Check sheet for the modelled part. Datum: model origin and axes. Units: mm. Face numbers are marked on the shaded views. Coordinates: 2 decimals unless noted, no trailing zeros. Loops run counter-clockwise (first coordinate to the right, second up) from the corner with the lowest first, then second, coordinate; pieces in that order, holes last. Notation, with made-up numbers: M 73,89 L 77,89 A16 ccw 77,103 Z; hole C 59,-2 d10. An arc over 180 degrees is marked long. Answer as CSV lines item,"result". Start each with the question number.
from build123d import *

# Parameters (mm, degrees)
F0_R     = 14.2875
F0_R_2   = 7.9375
F1_DEPTH = 4.7625
F2_R     = 1.190625
F3_DEPTH = 25.4
F5_DEPTH = 19.05


with BuildPart() as f1:
    # F0 (on Top) → F1 (new body)
    with BuildSketch(Plane.XY):
        Circle(F0_R)
        Circle(F0_R_2, mode=Mode.SUBTRACT)
    extrude(amount=F1_DEPTH)

    # F2 (on Top) → F3 (cut)
    with BuildSketch(Plane.XY):
        with Locations((0, 11.1125)):
            Circle(F2_R)
        with Locations((11.1125, 0)):
            Circle(F2_R)
        with Locations((-11.1125, 0)):
            Circle(F2_R)
        with Locations((0, -11.1125)):
            Circle(F2_R)
    extrude(amount=F3_DEPTH, mode=Mode.SUBTRACT)

    # F4 (on Top) → F5 (join)
    with BuildSketch(Plane.XY):
        with BuildLine():
            Line((5.61266, 5.61266), (12.347852, 12.347852))
            ThreePointArc((12.347852, 12.347852), (11.176734, 13.417135), (9.91344, 14.375765))
            Line((9.91344, 14.375765), (2.91897, 7.381295))
            ThreePointArc((2.91897, 7.381295), (4.356512, 6.635112), (5.61266, 5.61266))
        make_face()
        with BuildLine():
            Line((7.381295, 2.91897), (14.375765, 9.91344))
            ThreePointArc((14.375765, 9.91344), (13.417135, 11.176734), (12.347852, 12.347852))
            Line((12.347852, 12.347852), (5.61266, 5.61266))
            ThreePointArc((5.61266, 5.61266), (6.635112, 4.356512), (7.381295, 2.91897))
        make_face()
    extrude(amount=F5_DEPTH)


solid = f1.part
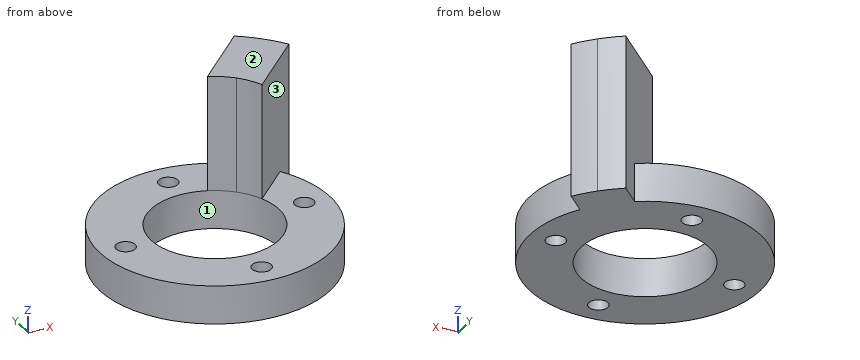
Item 1: Sectioned sample at B-B, the plane x = -3.5. Record the boundary of the cut face in (y, z).
Item 2: Release check for a two-part mould opening along X. For the marked faces 1, 2 and 3 record: released by +X, released by -X, zero draft, split by the parting line, or undercut.
Item 3: Material ranges on line 1 (X direction, y = 0, z = 1.3); line 2 (Z direction, x = -12.25, y = 0.75), recorded low to high. Write a range as from..to.
Item 4: Go/stop test with flat-tipped pins: pin 1 (2 mm diameter, centred on y = 6.5, z = 17, fed in from +X); pin 2 (1.9 mm diameter, centred on x = 0, y = 11.11, fed in from -Z); pin 3 (2 mm diameter, centred on y = 8, z = 5.5, fed in from +X); pin 4 (2.5 mm diameter, centred on x = 11.11, y = 0, fed in from +Z). Record where each tip stops, or that it passes through.
Item 5: Sectioned sample at D-D, the plane z = 15.5. Record the boundary of the cut face in (x, y).
Item 6: Sectioned sample at A-A, the plane y = 0. Record the boundary of the cut face in (x, z).
Reply:
1,outline,"M -13.85,0 L -7.12,0 L -7.12,4.76 L -13.85,4.76 Z; M 7.12,0 L 13.85,0 L 13.85,4.76 L 7.12,4.76 Z"
2,face 1,"undercut"
2,face 2,"zero draft"
2,face 3,"released by +X"
3,line 1,"-14.29..-12.3, -9.92..-7.94, 7.94..9.92, 12.3..14.29"
3,line 2,"0..4.76"
4,pin 1,"x = 11.96"
4,pin 2,"through"
4,pin 3,"x = 13.46"
4,pin 4,"z = 4.76"
5,outline,"M 2.92,7.38 A7.94 cw 5.61,5.61 A7.94 cw 7.38,2.92 L 14.38,9.91 A17.46 ccw 12.35,12.35 A17.46 ccw 9.91,14.38 Z"
6,outline,"M -14.29,0 L -12.3,0 L -12.3,4.76 L -14.29,4.76 Z; M -9.92,0 L -7.94,0 L -7.94,4.76 L -9.92,4.76 Z; M 7.94,0 L 9.92,0 L 9.92,4.76 L 7.94,4.76 Z; M 12.3,0 L 14.29,0 L 14.29,4.76 L 12.3,4.76 Z"
